Read the model definition and answer for the solid it produces. Units are mm, in the model's axes. Face numbers are marked on the shaded views. A direction names the side the tool comes from. Give positions to 0.01 mm unless a question says otherwise; leave off trailing zeros. Write each loop counter-clockwise with the first axis right and the second up, starting at its lowest first coordinate (ties: lowest second). Pieces come first, ordered by that corner, then holes.
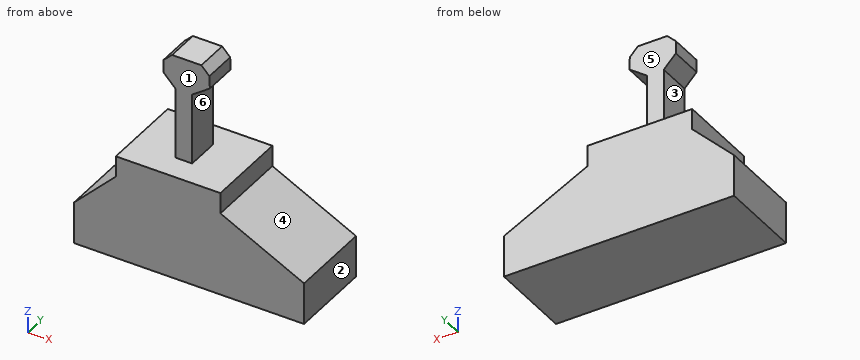
Autodesk Inventor part; units mm, degrees
ref_plane "YZ Plane" through (0, 0, 0) normal (1, 0, 0) x (0, 1, 0)
ref_plane "XZ Plane" through (0, 0, 0) normal (0, 1, 0) x (-1, 0, 0)
ref_plane "XY Plane" through (0, 0, 0) normal (0, 0, 1) x (1, 0, 0)
sketch "Эскиз1" plane through (0, 0, 0) normal (0, 0, 1) x (1, 0, 0)
  arc A0 (113.5, 24) -> (93.5, 4) centre (113.5, 4) ccw
  arc A1 (93.5, -1) -> (113.5, -21) centre (113.5, -1) ccw
  line L0 (93.5, 4) -> (93.5, -1)
  line L1 (88.5, 11.5) -> (28.5, 11.5)
  line L2 (28.5, 11.5) -> (28.5, -8.5)
  line L3 (28.5, -8.5) -> (88.5, -8.5)
  line L4 (88.5, -8.5) -> (88.5, 11.5)
  line L5 (-123.5, 102) -> (-123.5, -102)
  line L6 (-123.5, -102) -> (123.5, -102)
  line L7 (123.5, -102) -> (123.5, -100.4305)
  line L8 (123.5, -100.4305) -> (123.5, 102)
  line L9 (123.5, 102) -> (-123.5, 102)
  point P0 (0, 0)
  point P1 (88.5, 1.5)
  point P2 (93.5, 1.5)
  dimension "d0" = 20
  dimension "d1" = 60
  dimension "d2" = 5
extrude "Выдавливание1" add sketch "Эскиз1" along normal blind 30 contours L4 L3 L2 L1
sketch "Эскиз2" plane through (28.5, -8.5, 0) normal (0, -1, 0) x (1, 0, 0)
  line L0 (0, 0) -> (60, 0)
  line L1 (60, 0) -> (60, 3.0763)
  line L2 (60, 3.0763) -> (60, 10)
  line L3 (60, 10) -> (40, 20)
  line L4 (40, 20) -> (40, 25)
  line L5 (40, 25) -> (15, 25)
  line L6 (15, 25) -> (15, 20)
  line L7 (15, 20) -> (5, 10)
  line L8 (5, 10) -> (5, 0)
  line L9 (60, 0) -> (60, 30)
  point P0 (-28.5, 0)
  dimension "d6" = 25
  dimension "d7" = 5
  dimension "d8" = 5
  dimension "d9" = 20
  dimension "d10" = 10
  dimension "d11" = 10
  dimension "d12" = 10
  dimension "d13" = 25
extrude "Выдавливание2" cut sketch "Эскиз2" against normal blind 30 keep common part
sketch "Эскиз3" plane through (43.5, -8.5, 25) normal (0, 0, 1) x (1, 0, 0)
  line L0 (5, 14) -> (20, 14)
  line L1 (20, 14) -> (20, 6)
  line L2 (20, 6) -> (5, 6)
  line L3 (5, 6) -> (5, 14)
  line L4 (25, 20) -> (0, 20)
  line L5 (0, 0) -> (0, 20)
  point P0 (-43.5, 8.5)
  dimension "d16" = 8
  dimension "d17" = 15
  dimension "d18" = 6
  dimension "d19" = 25
  dimension "d20" = 20
  dimension "d21" = 5
extrude "Выдавливание3" add sketch "Эскиз3" along normal blind 25
sketch "Эскиз4" plane through (48.5, -2.5, 25) normal (0, -1, 0) x (1, 0, 0)
  line L0 (15, 0) -> (0, 0)
  line L1 (5.5312, 0) -> (5.5312, 17)
  line L2 (5.5312, 17) -> (2.6422, 20)
  line L3 (2.6422, 20) -> (2.6422, 23)
  line L4 (2.6422, 23) -> (4.719, 25)
  line L5 (4.719, 25) -> (11.719, 25)
  line L6 (0, 25) -> (15, 25)
  line L7 (11.719, 25) -> (13.645, 23)
  line L8 (13.645, 23) -> (13.7498, 20)
  line L9 (13.7498, 20) -> (9.5312, 17)
  line L10 (9.5312, 17) -> (9.5312, 0)
  line L11 (-5, 0) -> (20, 0)
  line L12 (0, 0) -> (0, 25)
  line L13 (5.5312, 0) -> (9.5312, 0)
  line L14 (20, -5) -> (40, -15)
  line L15 (20, 0) -> (20, -5)
  line L16 (-5, 0) -> (20, 0)
  line L17 (-5, -5) -> (-5, 0)
  line L18 (-15, -15) -> (-5, -5)
  line L19 (-15, -25) -> (-15, -15)
  line L20 (-15, -25) -> (40, -25)
  line L21 (40, -25) -> (40, -15)
  point P0 (-48.5, -25)
  point P1 (9.5312, 0)
  dimension "d24" = 2
  dimension "d25" = 7
  dimension "d26" = 17
  dimension "d27" = 17
  dimension "d28" = 3
  dimension "d29" = 3
  dimension "d30" = 3
  dimension "d31" = 3
  dimension "d32" = 2
  dimension "d33" = 4
  dimension "d34" = 11.1076
  dimension "d35" = 2.6422
extrude "Выдавливание4" cut sketch "Эскиз4" against normal through all both and the other way through all contours L11 L15 L14 L21 L20 L19 L18 L17 L0 | L0 L1 L2 L3 L4 L5 L7 L8 L9 L10 keep common part
equation "\"d18\" = -0.5 * d16 + 0.5 * d20"
equation "\"d21\" = -0.5 * d17 + 0.5 * d19"
properties part number "ДИ 00.00.06"
Item 1: Section C-C (z = 15) is taken. Write down the section's boundary in (x, y), and give its area (3 significant figures).
Result set:
outline: (38.5, -8.5) - (78.5, -8.5) - (78.5, 11.5) - (38.5, 11.5) - close
area: 800 mm2
Item 2: Section D-D (x = 73) is taken. Write down the section's boundary in (y, z), and give its area (3 significant figures).
Result set:
outline: (-8.5, 0) - (11.5, 0) - (11.5, 17.75) - (-8.5, 17.75) - close
area: 355 mm2
Item 3: Which of the six approach directions +Z, -Z, +X, -X, +Y, -Y give full straight-line access (tool end or side, diameter ignored) to the marked faces 1, 2 and 3?
Result set:
face 1: +Z, +X, -X, -Y
face 2: +Z, -Z, +X, +Y, -Y
face 3: -X, +Y, -Y
Item 4: Determine the mould class of the marked faces 4, 5 and 6 for opening direction Z: pulls with the +Z half, pulls with the -Z half, needs draft (parallel to the pull), parting line crosses it, or undercut.
Result set:
face 4: pulls with the +Z half
face 5: needs draft
face 6: undercut
Item 5: Section B-B (y = -3.75) is taken. Write down the section's boundary in (x, z).
Result set:
outline: (33.5, 0) - (88.5, 0) - (88.5, 10) - (68.5, 20) - (68.5, 25) - (43.5, 25) - (43.5, 20) - (33.5, 10) - close
Item 6: Each of these flat-tipped pins is pushed along its axis until it touches: pin 1 Ø2 at (x, y) = (47.5, 7.5) entering from +Z; pin 2 Ø6.5 at (y, z) = (2, 36.5) entering from +X; pin 3 Ø2.5 at (y, z) = (5, 22) entering from +X; pin 4 Ø1.5 at (y, z) = (-4, 43.5) entering from -X. Where does it stop, or does it pass through?
Result set:
pin 1: stops at z = 25
pin 2: stops at x = 58.03
pin 3: stops at x = 68.5
pin 4: passes through
Item 7: Find the intervals of material crossed by line 1 along Z through (x, y) = (56, 7.5); line 2 along X through (y, z) = (5, 13.5); line 3 along X through (y, z) = (4, 31), in increasing order.
Result set:
line 1: z = 0 to 25
line 2: x = 37 to 81.5
line 3: x = 54.03 to 58.03
Item 8: Section A-A (x = 59) is taken. Write down the section's boundary in (y, z).
Result set:
outline: (-8.5, 0) - (11.5, 0) - (11.5, 25) - (-8.5, 25) - close; (-2.5, 42.69) - (5.5, 42.69) - (5.5, 50) - (-2.5, 50) - close
